Check sheet for the modelled part. Datum: model origin and axes. Units: mm. A direction names the side the tool comes from. Coordinates: 2 decimals unless noted, no trailing zeros. Write each loop counter-clockwise with the first axis right and the second up, starting at its lowest first coordinate (ties: lowest second). Pieces come first, ordered by that corner, then holes. Notation, with made-up numbers: (63, 33.25) -> (69, 33.25) arc R26 cw to (69, 62.25) -> close; hole circle Ø9 at (15.5, -27). An arc over 180 degrees is marked (long way). One line per item, written item: value. Start each with the question number.
1) Sectioned sample at A-A on y = 698.5. Enter the section's corners in (x, z).
2) Sectioned sample at C-C on z = 19.5. Enter the section's corners in (x, y), plus the area to 3 significant figures.
3) Draft check along X on faces 3 (the flat face through (551.093, 460, 12)), 4 (the flat face through (-48.907, 474, 12)), 5 (the flat face through (51.093, 600, 12)), 6 (the cylindrical face through (254.086, 307.382, 12.325)). Enter one of: +X half, -X half, draft (parallel to the pull), parting line (faces both ways), or undercut.
4) Scan lines: line 1 along X through (y, z) = (919, 18.25); line 2 along Y through (x, z) = (214, 10); line 3 along Y through (x, z) = (177, 11.5). Record each from-to range of solid material in increasing order. Write a range as [from, to].
5) Set-up check for faces 1 (the flat face through (-19, -32.605, 12)), 2 (the flat face through (451.093, 610, 12)): record each of +Z, -Z, +X, -X, +Y, -Y from which the full face is reachable in a straight line by a thin tool's end or side.
6) Sectioned sample at D-D on y = 1181. Enter the section's corners in (x, z).
7) Gauge pin test, flat ends, axial feed: P1, Ø1, axis at x = 332.5, z = 19, coming from the +Y side; P2, Ø3, axis at x = 172, z = 3, coming from the +Y side; P3, Ø10, axis at x = 286.5, z = 8, coming from the +Y side. Record the tip position at first contact, or that the pin passes through.
8) Sectioned sample at B-B on x = 310. Enter the section's corners in (y, z).
```python
from build123d import *

# Parameters (mm, degrees)
F1_DEPTH = 25


with BuildPart() as f1:
    # F0 (on Top) → F1 (new body)
    with BuildSketch(Plane.XY):
        with BuildLine():
            Line((-48.90696, 967.395362), (-48.90696, -32.604638))
            Line((-48.90696, -32.604638), (11.09304, -32.604638))
            ThreePointArc((11.09304, -32.604638), (251.09304, 207.395362), (491.09304, -32.604638))
            Line((491.09304, -32.604638), (551.09304, -32.604638))
            Line((551.09304, -32.604638), (551.09304, 967.395362))
            ThreePointArc((551.09304, 967.395362), (251.09304, 1267.395362), (-48.90696, 967.395362))
        make_face()
        with BuildLine():
            Line((451.09304, 967.395362), (451.09304, 242.349903))
            ThreePointArc((451.09304, 242.349903), (251.09304, 307.395362), (51.09304, 242.349903))
            Line((51.09304, 242.349903), (51.09304, 967.395362))
            ThreePointArc((51.09304, 967.395362), (251.09304, 1167.395362), (451.09304, 967.395362))
        make_face(mode=Mode.SUBTRACT)
    extrude(amount=F1_DEPTH)


solid = f1.part
```
Answers:
1. outline: (-48.91, 0) -> (51.09, 0) -> (51.09, 25) -> (-48.91, 25) -> close; (451.09, 0) -> (551.09, 0) -> (551.09, 25) -> (451.09, 25) -> close
2. outline: (-48.91, -32.6) -> (11.09, -32.6) arc R240 cw to (491.09, -32.6) -> (551.09, -32.6) -> (551.09, 967.4) arc R300 ccw to (-48.91, 967.4) -> close; hole (51.09, 242.35) arc R340 cw to (451.09, 242.35) -> (451.09, 967.4) arc R200 ccw to (51.09, 967.4) -> close
2. area: 316,000 mm2
3. face 3: +X half
3. face 4: -X half
3. face 5: undercut
3. face 6: undercut
4. line 1: x = [-48.91, 51.09], [451.09, 551.09]
4. line 2: y = [204.51, 305.37], [1163.93, 1265.09]
4. line 3: y = [195.67, 299.22], [1153.16, 1258.1]
5. face 1: +Z, -Z, +X, -X, -Y
5. face 2: +Z, -Z
6. outline: (40.44, 0) -> (461.74, 0) -> (461.74, 25) -> (40.44, 25) -> close
7. P1: stops at y = 1256.28
7. P2: stops at y = 1257.19
7. P3: stops at y = 1265.85
8. outline: (200.05, 0) -> (302.25, 0) -> (302.25, 25) -> (200.05, 25) -> close; (1158.52, 0) -> (1261.56, 0) -> (1261.56, 25) -> (1158.52, 25) -> close
